The model under review builds one solid part; all positions refer to its coordinate system, in mm. Face numbers are marked on the shaded views. A direction names the side the tool comes from. Give positions to 0.01 mm unless a question says otherwise; leave off trailing zeros. Write each loop counter-clockwise with the first axis right and the second up, starting at its lowest first coordinate (ties: lowest second). Pieces come first, ordered by that corner, then holes. Notation, with made-up numbers: (-3, 43) - (29, 43) arc R12 cw to (29, 57) - close; hole circle Ø10 at (-2.5, 32.25). An arc over 180 degrees is marked (long way). One line per question, with ' | ' between items. Start each with the question number.
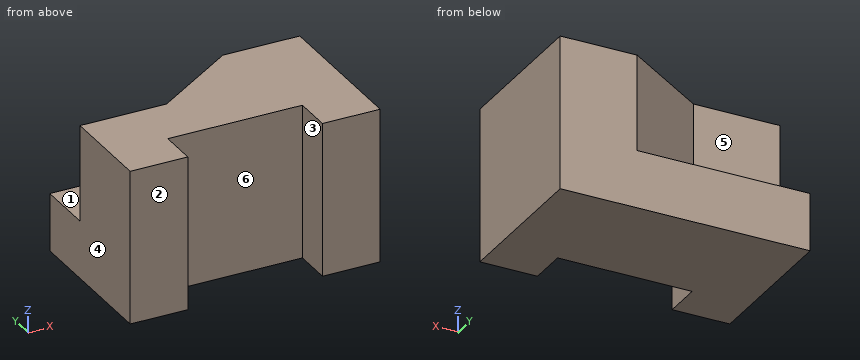
```python
from build123d import *

# Parameters (mm, degrees)
BOSS_EXTRUDE1_DEPTH = 8
CUT_EXTRUDE1_DEPTH  = 5


with BuildPart() as part:
    # Sketch1 → Boss-Extrude1 (new body)
    with BuildSketch(Plane.XY):
        Polygon((0, 8), (0, 0), (3, 0), (3, 2), (10, 2), (10, 0), (13, 0), (13, 8), align=None)
    extrude(amount=BOSS_EXTRUDE1_DEPTH)

    # Sketch2 → Cut-Extrude1 (cut)
    with BuildSketch(Plane.XY.offset(8)):
        Polygon((9, 8), (4.5, 5), (0, 5), (0, 8), align=None)
    extrude(amount=-CUT_EXTRUDE1_DEPTH, mode=Mode.SUBTRACT)


solid = part.part
```
Item 1: Machinability: for the marked faces 1, 2 and 3, which of the approach directions +Z, -Z, +X, -X, +Y, -Y give a long, thin tool a straight path to every point of the face, cutting with its end or side? Answer none if there is none.
Item 2: The part is to be moulded in two halves that separate along X. For the marked faces 4, 5 and 6, say which applies: +X half, -X half, draft (parallel to the pull), parting line (faces both ways), or undercut.
Item 3: Take a section at C-C (x = 6). Give the boundary of the cut face in (y, z).
Item 4: For probe 1 along X at (y, z) = (1.5, 1.5); probe 2 along Y at (x, z) = (3.25, 1.25); probe 3 along Y at (x, z) = (3.5, 6.5), list the stretches that pass through material, from the lowest coordinate up.
Item 5: Take a section at B-B (z = 6). Give the boundary of the cut face in (x, y), plus the area to 4 significant figures.
Item 6: Clearance check with flat-ended pins moving along their axes: P1, Ø1.6, axis at y = 1, z = 6, coming from the -X side; P2, Ø3.5, axis at x = 2.5, z = 5.5, coming from the +Y side. State where each tip first meets the part, or that it passes through.
Item 7: Take a section at A-A (y = 1.5). Give the boundary of the cut face in (x, z).
Item 8: Take a section at D-D (y = 6.5). Give the boundary of the cut face in (x, z).
Check sheet entries:
1) face 1: +Z, -X, +Y | face 2: +Z, -Z, +X, -X, -Y | face 3: +Z, -Z, -Y
2) face 4: -X half | face 5: draft | face 6: undercut
3) outline: (2, 0) - (8, 0) - (8, 3) - (6, 3) - (6, 8) - (2, 8) - close
4) probe 1: x = 0 to 3, 10 to 13 | probe 2: y = 2 to 8 | probe 3: y = 2 to 5
5) outline: (0, 0) - (3, 0) - (3, 2) - (10, 2) - (10, 0) - (13, 0) - (13, 8) - (9, 8) - (4.5, 5) - (0, 5) - close | area: 69.75 mm^2
6) P1: stops at x = 0 | P2: stops at y = 5
7) outline: (0, 0) - (3, 0) - (3, 8) - (0, 8) - close; (10, 0) - (13, 0) - (13, 8) - (10, 8) - close
8) outline: (0, 0) - (13, 0) - (13, 8) - (6.75, 8) - (6.75, 3) - (0, 3) - close
